```python
from build123d import *

# Parameters (mm, degrees)
BOSS_EXTRUDE1_DEPTH       = 30
FILLET1_R                 = 4
FILLET2_R                 = 4
F_3_0MM_DOWEL_HOLE1_D     = 3
F_3_0MM_DOWEL_HOLE1_DEPTH = 2
F_3_0MM_DOWEL_HOLE2_D     = 3
F_3_0MM_DOWEL_HOLE2_DEPTH = 2


with BuildPart() as part:
    # Sketch1 → Boss-Extrude1 (new body)
    with BuildSketch(Plane.XY):
        Polygon((0, 0), (25, 0), (25, -2), (-2, -2), (-2, 25), (0, 25), align=None)
    extrude(amount=-BOSS_EXTRUDE1_DEPTH)

    # Fillet1
    fillet1_edges = [part.edges().sort_by_distance(p)[0] for p in [
        (0, 0, -15),
    ]]
    fillet(fillet1_edges, radius=FILLET1_R)

    # Fillet2
    fillet2_edges = [part.edges().sort_by_distance(p)[0] for p in [
        (-2, -2, -15),
    ]]
    fillet(fillet2_edges, radius=FILLET2_R)

    # Ø3.0mm Dowel Hole1
    with Locations(Plane(origin=(0, 0, 0), x_dir=(1, 0, 0), z_dir=(0, 1, 0))):
        with Locations((14.5, 22.5), (14.5, 7.5)):
            Hole(F_3_0MM_DOWEL_HOLE1_D / 2, depth=F_3_0MM_DOWEL_HOLE1_DEPTH)

    # Ø3.0mm Dowel Hole2
    with Locations(Plane(origin=(0, 0, 0), x_dir=(0, 0, -1), z_dir=(1, 0, 0))):
        with Locations((7.5, 14.5), (22.5, 14.5)):
            Hole(F_3_0MM_DOWEL_HOLE2_D / 2, depth=F_3_0MM_DOWEL_HOLE2_DEPTH)


solid = part.part
```
Read the model definition and answer for the solid it produces. Units are mm, in the model's axes. A direction names the side the tool comes from. Round coordinates to 2 decimals unless told otherwise and drop trailing zeros. Write each loop counter-clockwise with the first axis right and the second up, starting at its lowest first coordinate (ties: lowest second). Pieces come first, ordered by that corner, then holes. Notation, with made-up numbers: (58, 65.5) - (75, 65.5) arc R21 ccw to (75, 79.5) - close; hole circle Ø1 at (69.25, 45.25). An arc over 180 degrees is marked (long way). One line per item, written item: value.
Q1. Which of the six approach directions +Z, -Z, +X, -X, +Y, -Y give full straight-line access (tool end or side, diameter ignored) to faces 1 (the flat face through (14, 0, -15)), 2 (the cylindrical face through (15.7, -1, -6.6))?
The answers:
face 1: +Z, -Z, +X, +Y
face 2: +Y, -Y
Q2. Find section A-A (y = 14.5). Determine the outline of the cut face in (x, z), and give its area (3 significant figures).
The answers:
outline: (-2, -30) - (0, -30) - (0, -24) - (-2, -24) - close; (-2, -21) - (0, -21) - (0, -9) - (-2, -9) - close; (-2, -6) - (0, -6) - (0, 0) - (-2, 0) - close
area: 48.0 mm2
Q3. Each of these flat-tipped pins is pushed along its axis until it touches: P1, Ø10.5, axis at x = 12, z = -17.5, coming from the +Y side; P2, Ø4, axis at y = 14.5, z = -7.5, coming from the +X side. Where does it stop, or does it pass through?
The answers:
P1: stops at y = 0
P2: stops at x = 0
Q4. Find section D-D (z = -17.75). Determine the outline of the cut face in (x, y).
The answers:
outline: (-2, 2) arc R4 ccw to (2, -2) - (25, -2) - (25, 0) - (4, 0) arc R4 cw to (0, 4) - (0, 25) - (-2, 25) - close
Q5. For a pull along Z with two mould halves and no side action, classify faces 3 (the cylindrical face through (-1.01, 14.57, -24)), 4 (the cylindrical face through (1.203, 1.141, -15.21)), 5 (the cylindrical face through (15.61, -1.01, -23.51)), 6 (the flat face through (5.6, -0.4, 0)) as pulls with the +Z half, pulls with the -Z half, needs draft (parallel to the pull), parting line crosses it, or undercut.
The answers:
face 3: undercut
face 4: needs draft
face 5: undercut
face 6: pulls with the +Z half
Q6. Find section B-B (z = -22.5). Determine the outline of the cut face in (x, y).
The answers:
outline: (-2, 2) arc R4 ccw to (2, -2) - (13, -2) - (13, 0) - (4, 0) arc R4 cw to (0, 4) - (0, 13) - (-2, 13) - close; (-2, 16) - (0, 16) - (0, 25) - (-2, 25) - close; (16, -2) - (25, -2) - (25, 0) - (16, 0) - close
Q7. Straight lines are drawn through the part: line 1 (Z direction, x = 14.5, y = -0.65); line 2 (Y direction, x = 13.5, z = -21). For each, find the intervals that lie inside material, in ascending order. Write a range as from..to.
The answers:
line 1: z = -30..-24, -21..-9, -6..0
line 2: y = -2..0
